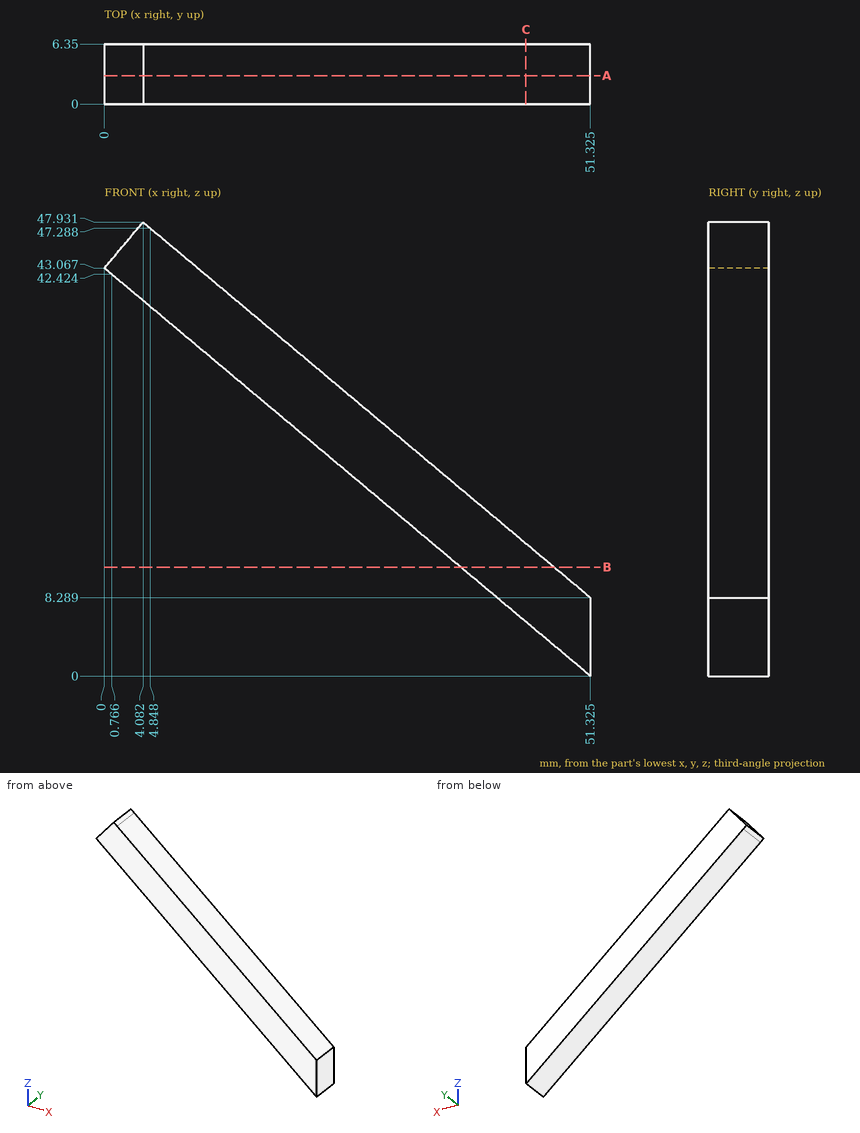
For this review, use the dimensioned drawing (mm, ordinates from the lowest corner) and the shaded views. Coordinates: 2 decimals unless noted, no trailing zeros. Order: outer loops, then holes, each group sorted by start corner. A loop starts at its lowest first (then second) coordinate and runs counter-clockwise, first axis right, second up. Notation, with made-up numbers: M 77,-2.5 L 101,-2.5 A8 ccw 101,6.5 Z; hole C -20.75,75.5 d9. An arc over 180 degrees is marked long. Answer as a JSON object with one key per item and string values. Group by question number.
1) Wall thickness on L1, parallel to X at y = 0.5, z = 10 (1 decimal); L2, parallel to X at y = 2.75, z = 15.5 (1 decimal); L3, parallel to Z at x = 35.5, y = 1: over which ranges is each line inside the solid? List them lowest first.
2) Add section A-A, the plane y = 3. Write out the cut boundary in (x, z) (1 decimal).
3) Add section C-C, the plane x = 44.5. Write out the cut boundary in (y, z).
4) For pin 1 (2 mm diameter, centred on x = 38.5, y = 2.5, fed in from -Z); pin 2 (1 mm diameter, centred on x = 44.5, y = 5.5, fed in from +Z) (1 decimal), all flat-tipped, find the tip position at first contact; note any pin that passes through.
5) Add section B-B, the plane z = 11.5. Write out the cut boundary in (x, y).
Computed values:
{
 "1": {"L1": "x = 39.4 to 49.3", "L2": "x = 32.9 to 42.7", "L3": "z = 13.28 to 21.57"},
 "2": {"outline": "M 0,43.1 L 0.8,42.4 L 51.3,0 L 51.3,8.3 L 4.8,47.3 L 4.1,47.9 Z"},
 "3": {"outline": "M 0,5.73 L 6.35,5.73 L 6.35,14.02 L 0,14.02 Z"},
 "4": {"pin 1": "stops at z = 9.92", "pin 2": "stops at z = 14.4"},
 "5": {"outline": "M 37.62,0 L 47.5,0 L 47.5,6.35 L 37.62,6.35 Z"}
}
